Model file for the job. Use its own axes, mm. Face numbers are marked on the shaded views. Coordinates: 2 decimals unless noted, no trailing zeros. Write each loop counter-clockwise with the first axis right and the second up, starting at its lowest first coordinate (ties: lowest second). Pieces come first, ordered by that corner, then holes.
Q1. Band-saw the part on C-C, the plane z = -31. Write the cut outline in (x, y).
Q2. Band-saw the part on A-A, the plane x = -21. State how many separate pieces and enclosed holes the cut face has, plus the area to 3 significant figures.
Q3. Pull direction Z, two halves, no side cores. Call the marked faces 1, 2 and 3: released by +Z, released by -Z, zero draft, split by the parting line, or undercut.
Q4. Band-saw the part on D-D, the plane x = -36.5. Write the cut outline in (y, z).
Q5. Band-saw the part on B-B, the plane z = -23.5. Write the cut outline in (x, y).
Q6. Drill centre lines: probe 1 along X at (y, z) = (3.6, -8.2); probe 2 along X at (y, z) = (7.25, -40.5). Where is each one in solid material? Low to high.
Q7. Pin check, flat tips, straight feed: P1, Ø5, axis at x = -41.8, z = -8.2, coming from the +Y side; P2, Ø1.5, axis at x = -40, y = 3, coming from the +Z side; P3, Ø4.5, axis at y = 1.5, z = -24.5, coming from the -X side. Stop position of each tip, or through.
Autodesk Inventor part; units mm, degrees
ref_plane "YZ Plane" through (0, 0, 0) normal (1, 0, 0) x (0, 1, 0)
ref_plane "XZ Plane" through (0, 0, 0) normal (0, 1, 0) x (-1, 0, 0)
ref_plane "XY Plane" through (0, 0, 0) normal (0, 0, 1) x (1, 0, 0)
sketch "Sketch1" plane through (0, 0, 0) normal (0, 1, 0) x (-1, 0, 0)
  line L0 (0, 0) -> (50, 0)
  line L1 (50, 0) -> (50, -50)
  line L2 (50, -50) -> (0, -50)
  line L3 (0, -50) -> (0, 0)
  dimension "d0" = 50
  dimension "d1" = 50
extrude "Extrusion1" add sketch "Sketch1" along normal blind 7.5
fillet "Fillet1" radius 5 4 edges at (-50, 3.75, 0) (-50, 3.75, -50) (0, 3.75, -50) (0, 3.75, 0)
ref_plane "Work Plane2" through (-25, 7.5, -50) normal (-1, 0, 0) x (0, -1, 0)
ref_plane "Work Plane1" through (0, 7.5, -25) normal (0, 0, -1) x (-1, 0, 0)
fillet "Fillet2" radius 5 8 edges at (-1.4645, 0, -48.5355) (-25, 0, -50) (-48.5355, 0, -48.5355) (-50, 0, -25) (-48.5355, 0, -1.4645) (-25, 0, 0) (-1.4645, 0, -1.4645) (0, 0, -25)
shell "Shell1" thickness 4 removed faces 1 at (-16.6667, 7.5, -18.3333)
sketch "Sketch2" plane through (0, 0, 0) normal (0, -1, 0) x (1, 0, 0)
  line L0 (-25, -60) -> (-25, 10)
  line L1 (10, -25) -> (-60, -25)
  line L2 (-8.2, -8.2) -> (-41.8, -8.2) construction
  line L3 (-41.8, -8.2) -> (-41.8, -41.8) construction
  line L4 (-41.8, -41.8) -> (-8.2, -41.8) construction
  line L5 (-8.2, -41.8) -> (-8.2, -8.2) construction
  circle A0 centre (-8.2, -8.2) radius 1.5
  point P0 (0, 0)
  point P1 (-5, -45)
  point P2 (-45, -45)
  point P3 (-25, -41.8)
  point P4 (-8.2, -25)
  point P5 (-8.2, -25)
  point P6 (-25, -41.8)
  dimension "d8" = 33.6
  dimension "d9" = 33.6
  dimension "d10" = 3
extrude "Extrusion2" cut sketch "Sketch2" against normal up to surface (4 mm away)
ref_plane "Work Plane3" through (-8.2, 0, -8.2) normal (-1, 0, 0) x (0, -1, 0)
sketch "Sketch3" plane through (-8.2, 0, -8.2) normal (-1, 0, 0) x (0, -1, 0)
  line L0 (-4, -1.5) -> (-4, 1.5)
  line L1 (0, 1.5) -> (0, -1.5)
  line L2 (0, -36.8) -> (0, 3.2)
  line L3 (0, 2.75) -> (-1.5, 2.75)
  line L4 (-1.5, 2.75) -> (-1.5, -2.75)
  line L5 (-1.5, -2.75) -> (0, -2.75)
  line L6 (0, -2.75) -> (0, 2.75)
  line L7 (-1.5, -2.75) -> (-2.5, -1.5)
  line L8 (0, -1.5) -> (-4, -1.5)
  line L9 (0, 0) -> (-4, 0)
  point P0 (0, 8.2)
  point P1 (0, -2.75)
  dimension "d13" = 5.5
  dimension "d14" = 1.5
  dimension "d15" = 1
revolve "Revolution1" cut sketch "Sketch3" angle 360 about axis through (-8.2, 0, -8.2) along (0, 1, 0) contours L8 L4 L7 | L4 L8 L2 L5
mirror "Mirror1" about plane through (0, 7.5, -25) normal (0, 0, -1) of "Extrusion2", "Revolution1"
mirror "Mirror2" about plane through (-25, 7.5, -50) normal (-1, 0, 0) of "Extrusion2", "Mirror1", "Revolution1"
sketch "Sketch4" plane through (-45, 4, -45) normal (0, 1, 0) x (1, 0, 0)
  line L0 (20, -55) -> (20, 15) construction
  line L1 (-15, -20) -> (55, -20) construction
  line L2 (24, -23.2) -> (24, -16.8) construction
  line L3 (25.8, -23.2) -> (25.8, -16.8)
  line L4 (22.2, -16.8) -> (22.2, -23.2)
  arc A0 (22.2, -23.2) -> (25.8, -23.2) centre (24, -23.2) ccw
  arc A1 (25.8, -16.8) -> (22.2, -16.8) centre (24, -16.8) ccw
  point P0 (45, -45)
  point P1 (24, -20)
  point P2 (24, -15)
  point P3 (24, -25)
  dimension "d17" = 3.6
  dimension "d38" = 6.4
  dimension "d39" = 4
extrude "Extrusion3" cut sketch "Sketch4" against normal up to surface (4 mm away)
ref_plane "Płaszczyzna konstrukcyjna9" through (-19.09, 4, -28.2) normal (-1, 0, 0) x (0, 0, 1)
sketch "Szkic6" plane through (-19.09, 4, -28.2) normal (-1, 0, 0) x (0, 0, 1)
  line L0 (0, 0) -> (0, 0)
  line L1 (0, 0) -> (6.4, 0)
  line L2 (6.4, 0) -> (6.4, 0)
  line L3 (6.4, 0) -> (0, 0)
  line L4 (-15.1, 0) -> (-12.1, 0)
  line L5 (18.5, 0) -> (21.5, 0)
  line L6 (-15.1, 0) -> (-12.1, 0)
  line L7 (18.5, 0) -> (21.5, 0)
  line L8 (23.2, 0) -> (-16.8, 0)
  line L9 (-16.8, 0) -> (23.2, 0)
  line L10 (6.4, -4) -> (6.4, -4)
  line L11 (6.4, 0) -> (6.4, -4)
  line L12 (6.4, 0) -> (6.4, 0)
  line L13 (6.4, 0) -> (6.4, -4)
  line L14 (0, -4) -> (0, -4)
  line L15 (0, 0) -> (0, -4)
  line L16 (0, 0) -> (0, 0)
  line L17 (0, 0) -> (0, -4)
  line L18 (-16.55, 0) -> (-10.05, 0)
  line L19 (-10.05, 0) -> (-10.05, 6.85)
  line L20 (-10.05, 6.85) -> (-16.55, 6.85)
  line L21 (-16.55, 6.85) -> (-16.55, 0)
  circle A0 centre (-13.3, 3.6) radius 1.25
  line L22 (-13.3, 0) -> (-13.3, 6.85) construction
  line L23 (3.2, -6.17) -> (3.2, 9.02) construction
  line L24 (22.95, 0) -> (16.45, 0)
  line L25 (16.45, 0) -> (16.45, 6.85)
  line L26 (16.45, 6.85) -> (22.95, 6.85)
  line L27 (22.95, 6.85) -> (22.95, 0)
  circle A1 centre (19.7, 3.6) radius 1.25
  line L28 (19.7, 0) -> (19.7, 6.85) construction
  point P0 (28.2, -4)
  point P1 (16.45, 0)
  point P2 (18.5, 0)
  point P3 (21.5, 0)
  point P4 (-16.55, 0)
  point P5 (-15.1, 0)
  point P6 (-12.1, 0)
  point P7 (-10.05, 0)
  dimension "d30" = 2
  dimension "d31" = 2
  dimension "d33" = 3.6
  dimension "d34" = 2.5
  dimension "d35" = 33
extrude "Wyciągnięcie proste5" add sketch "Szkic6" along normal blind 6
fillet "Zaokrąglenie3" radius 2 4 edges at (-22.09, 10.85, -38.25) (-22.09, 10.85, -44.75) (-22.09, 10.85, -11.75) (-22.09, 10.85, -5.25)
equation "\"d0\" = blob_overall"
equation "\"d1\" = blob_overall"
equation "\"d4\" = corner_round"
equation "\"d5\" = corner_round"
equation "\"d6\" = shell_width"
equation "\"d31\" = d30"
equation "\"blob_overall\" = 50"
equation "\"corner_round\" = 5"
equation "\"matrix_size\" = 32"
equation "\"shell_width\" = 4"
properties part number "case2"
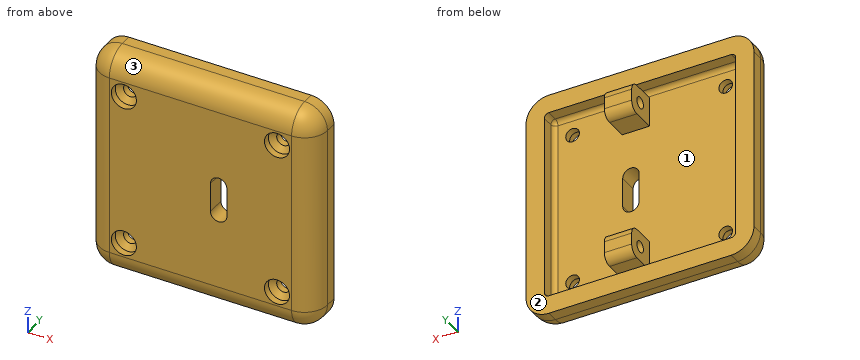
Answer sheet:
1. outline: (-50, 5) arc R5 ccw to (-45, 0) - (-5, 0) arc R5 ccw to (0, 5) - (0, 7.5) - (-4, 7.5) - (-4, 5) arc R1 cw to (-5, 4) - (-45, 4) arc R1 cw to (-46, 5) - (-46, 7.5) - (-50, 7.5) - close
2. separate pieces: 2
2. enclosed holes: 2
2. area: 253 mm2
3. face 1: undercut
3. face 2: zero draft
3. face 3: released by +Z
4. outline: (0, -45) arc R5 ccw to (5, -50) - (7.5, -50) - (7.5, -46) - (5, -46) arc R1 cw to (4, -45) - (4, -5) arc R1 cw to (5, -4) - (7.5, -4) - (7.5, 0) - (5, 0) arc R5 ccw to (0, -5) - close
5. outline: (-50, 5) arc R5 ccw to (-45, 0) - (-22.8, 0) - (-22.8, 4) - (-45, 4) arc R1 cw to (-46, 5) - (-46, 7.5) - (-50, 7.5) - close; (-19.2, 0) - (-5, 0) arc R5 ccw to (0, 5) - (0, 7.5) - (-4, 7.5) - (-4, 5) arc R1 cw to (-5, 4) - (-19.2, 4) - close
6. probe 1: x = -49.8 to -43.3, -40.3 to -9.7, -6.7 to -0.2
6. probe 2: x = -50 to -46, -4 to 0
7. P1: stops at y = 4
7. P2: stops at z = -0.16
7. P3: stops at x = -49.84
